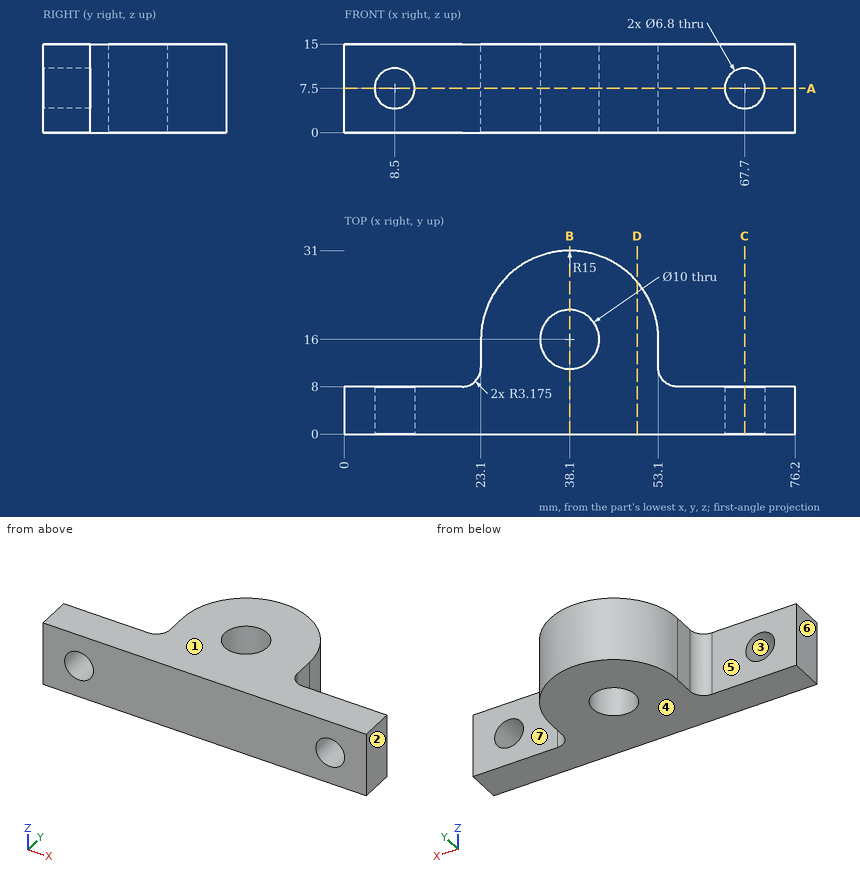
The drawing under review shows one solid part. Ordinate dimensions are in mm from its lowest x, y, z. A direction names the side the tool comes from. Give positions to 0.01 mm unless a question says otherwise; leave off trailing zeros. Order: outer loops, then holes, each group sorted by start corner. A loop starts at its lowest first (then second) coordinate and runs counter-clockwise, first axis right, second up. Notation, with made-up numbers: M -28,83 L 20,83 A28 ccw 20,109 Z; hole C 64,84 d1. An arc over 180 degrees is marked long. Answer in a Markdown table with one row per item. Add a question column.
1. For pin 1 Ø1.4 at (y, z) = (14.5, 6.5) entering from -X; pin 2 Ø4 at (y, z) = (12.5, 8.5) entering from +X; pin 3 Ø2 at (y, z) = (19.5, 4.5) entering from -X, all flat-tipped, find the tip position at first contact; note any pin that passes through.
2. Add section D-D on x = 49.5. State the section outline as (y, z) points.
3. Add section C-C on x = 67.7. State the section outline as (y, z) points, plus the area to 3 significant figures.
4. Mouldability with a two-part tool opening along Z and no side actions: class the marked faces 1, 2, 3 and 4 as released by +Z, released by -Z, zero draft, split by the parting line, or undercut.
5. To check wall thickness, follow line 1 along Y through (x, z) = (38.1, 9.25); line 2 along Y through (x, z) = (13, 2.25); line 3 along Z through (x, y) = (67, 4). State the ranges of each line that lie inside material, in increasing order.
6. Add section A-A on z = 7.5. State the section outline as (x, y) points (3 decimals).
7. Machinability: for the marked faces 5, 6 and 7, which of the approach directions +Z, -Z, +X, -X, +Y, -Y give a long, thin tool a straight path to every point of the face, cutting with its end or side? Answer none if there is none.
8. Add section B-B on x = 38.1. State the section outline as (y, z) points.
The answers:
| question | item | result |
|---|---|---|
| 1 | pin 1 | x = 23.1 |
| 1 | pin 2 | x = 53.17 |
| 1 | pin 3 | x = 23.31 |
| 2 | outline | M 0,0 L 25.75,0 L 25.75,15 L 0,15 Z |
| 3 | outline | M 0,0 L 8,0 L 8,4.1 L 0,4.1 Z; M 0,10.9 L 8,10.9 L 8,15 L 0,15 Z |
| 3 | area | 65.6 mm2 |
| 4 | face 1 | released by +Z |
| 4 | face 2 | zero draft |
| 4 | face 3 | undercut |
| 4 | face 4 | released by -Z |
| 5 | line 1 | 0 to 11, 21 to 31 |
| 5 | line 2 | 0 to 8 |
| 5 | line 3 | 0 to 4.17, 10.83 to 15 |
| 6 | outline | M 0,0 L 5.1,0 L 5.1,8 L 0,8 Z; M 11.9,0 L 64.3,0 L 64.3,8 L 56.275,8 A3.175 cw 53.1,11.175 L 53.1,16 A15 ccw 23.1,16 L 23.1,11.175 A3.175 cw 19.925,8 L 11.9,8 Z; M 71.1,0 L 76.2,0 L 76.2,8 L 71.1,8 Z; hole C 38.1,16 d10 |
| 7 | face 5 | +Z, -Z, -X, +Y |
| 7 | face 6 | +Z, -Z, -X, +Y, -Y |
| 7 | face 7 | +Z, -Z, +X, +Y |
| 8 | outline | M 0,0 L 11,0 L 11,15 L 0,15 Z; M 21,0 L 31,0 L 31,15 L 21,15 Z |
